Geometry: final body of the model. Coordinates: model frame, mm. A direction names the side the tool comes from. Round coordinates to 2 decimals unless told otherwise and drop trailing zeros. Order: outer loops, then holes, each group sorted by start corner. A loop starts at its lowest first (then second) coordinate and runs counter-clockwise, first axis right, second up. Notation, with made-up numbers: (56, -29.5) - (90, -29.5) arc R5 ccw to (90, -25.5) - close; hole circle Ø6 at (41, 68). An arc over 180 degrees is marked (long way). Put each result on its own line as item: value. Start each with the question number.
(1) Section C-C (y = 0). Output: boundary loops of the cut face in (x, z).
(2) Section A-A (z = -16). Output: boundary loops of the cut face in (x, y).
(3) Section B-B (x = 54). Output: boundary loops of the cut face in (y, z).
(4) Pull-direction query (Y, two-part tool) for faces 6 (the face through (67, 0, -10)), 7 (the face through (72, -9.1, -10)), 8 (the face through (33, 5, -1)); classes: released by +Y, released by -Y, zero draft, split by the parting line, or undercut.
(5) Section D-D (z = -13). Output: boundary loops of the cut face in (x, y).
(6) Access query for faces 1 (the face through (72, 9.1, -10)), 2 (the face through (34, -5, -1)), 3 (the face through (32, 2, -2)), 4 (the face through (71, 11.1, -10)), 5 (the face through (32, 1.75, -1)). Directions: +Z, -Z, +X, -X, +Y, -Y. A direction counts if a zero-diameter tool reaches every point of the face in a straight line with its end or side. Return the directions, or none.
(7) Material intervals for L1, parallel to Y at x = 68.65, z = -16; L2, parallel to X at y = -5.75, z = -5; L3, parallel to Z at x = 4.5, y = 2.25, sorted ascending. Write a range as [from, to].
(8) Pin query (flat end, axial travel): P1, Ø2, axis at x = 28.5, z = -0.5, coming from the -Y side; P2, Ø8, axis at x = 13.5, y = 2, coming from the -Z side; P3, Ø10, axis at y = 0.5, z = -10.5, coming from the -X side; P4, Ø10, axis at y = 0.5, z = -5.5, coming from the -X side. Return the tip coordinate at first contact, or that it passes through.
from build123d import *

# Parameters (mm, degrees)
BOSS_EXTRUDE1_DEPTH = 2
BOSS_EXTRUDE2_DEPTH = 20
SKETCH3_R           = 1.8
CUT_EXTRUDE1_DEPTH  = 15


with BuildPart() as part:
    # Sketch1 → Boss-Extrude1 (new body)
    with BuildSketch(Plane.XY):
        with BuildLine():
            Line((0, 5), (70, 5))
            Line((70, 5), (70, -5))
            Line((70, -5), (0, -5))
            ThreePointArc((0, -5), (-5, 0), (0, 5))
        make_face()
        with BuildLine():
            Line((0, 1.75), (65, 1.75))
            ThreePointArc((65, 1.75), (66.75, 0), (65, -1.75))
            Line((65, -1.75), (0, -1.75))
            ThreePointArc((0, -1.75), (-1.75, 0), (0, 1.75))
        make_face(mode=Mode.SUBTRACT)
    extrude(amount=-BOSS_EXTRUDE1_DEPTH)

    # Sketch2 → Boss-Extrude2 (add)
    with BuildSketch(Plane.XY):
        Polygon((74, 11.1), (67, 11.1), (67, -11.1), (74, -11.1), (74, -9.1), (70, -9.1), (70, 9.1), (74, 9.1), align=None)
    extrude(amount=-BOSS_EXTRUDE2_DEPTH)

    # Sketch3 → Cut-Extrude1 (cut)
    with BuildSketch(Plane.ZY.offset(-67)):
        with Locations((-16, 0)):
            Circle(SKETCH3_R)
    extrude(amount=-CUT_EXTRUDE1_DEPTH, mode=Mode.SUBTRACT)


solid = part.part
Checks:
1. outline: (-5, -2) - (-1.75, -2) - (-1.75, 0) - (-5, 0) - close; (66.75, -2) - (67, -2) - (67, -14.2) - (70, -14.2) - (70, 0) - (66.75, 0) - close; (67, -20) - (70, -20) - (70, -17.8) - (67, -17.8) - close
2. outline: (67, -11.1) - (74, -11.1) - (74, -9.1) - (70, -9.1) - (70, -1.8) - (67, -1.8) - close; (67, 1.8) - (70, 1.8) - (70, 9.1) - (74, 9.1) - (74, 11.1) - (67, 11.1) - close
3. outline: (-5, -2) - (-1.75, -2) - (-1.75, 0) - (-5, 0) - close; (1.75, -2) - (5, -2) - (5, 0) - (1.75, 0) - close
4. face 6: zero draft
4. face 7: undercut
4. face 8: released by +Y
5. outline: (67, -11.1) - (74, -11.1) - (74, -9.1) - (70, -9.1) - (70, 9.1) - (74, 9.1) - (74, 11.1) - (67, 11.1) - close
6. face 1: +Z, -Z, +X
6. face 2: +Z, -Z, -X, -Y
6. face 3: -Z, -X, +Y, -Y
6. face 4: +Z, -Z, +X, -X, +Y
6. face 5: +Z, -Z
7. L1: y = [-11.1, -1.8], [1.8, 11.1]
7. L2: x = [67, 70]
7. L3: z = [-2, 0]
8. P1: stops at y = -5
8. P2: stops at z = -2
8. P3: stops at x = 67
8. P4: stops at x = -5
